```python
from build123d import *

# Parameters (mm, degrees)
SKETCH1_W                = 304.8
SKETCH1_H                = 304.8
BOSS_EXTRUDE1_DEPTH      = 5.334
SKETCH2_W                = 6.35
SKETCH2_H                = 101.6
CUT_EXTRUDE1_DEPTH       = 216.592141684
SKETCH26_W               = 11.599333334
SKETCH26_H               = 5.334
SKETCH26_W_2             = 5.334
SKETCH26_H_2             = 19.05
CUT_EXTRUDE11_DEPTH      = 216.592141684
SKETCH27_W               = 11.599333334
SKETCH27_H               = 5.334
SKETCH27_W_2             = 5.334
SKETCH27_H_2             = 19.05
CUT_EXTRUDE12_DEPTH      = 216.592141684
SKETCH29_W               = 304.8
SKETCH29_H               = 24.084758951
CUT_EXTRUDE13_DEPTH      = 216.592141684
SKETCH31_R               = 1.374999997
CUT_EXTRUDE15_DEPTH      = 216.592141684
SKETCH32_R               = 1.25
CUT_EXTRUDE16_DEPTH      = 216.592141684
SKETCH34_R               = 1.249249953
SKETCH34_R_2             = 1.249999995
SKETCH34_R_3             = 1.252496274
SKETCH34_R_4             = 1.251959019
CUT_EXTRUDE18_DEPTH      = 216.592141684
SKETCH38_R               = 1.248199844
SKETCH38_R_2             = 1.253619174
SKETCH38_R_3             = 1.25252158
SKETCH38_R_4             = 1.237868742
CUT_EXTRUDE22_DEPTH      = 216.592141684
SKETCH40_W               = 304.8
SKETCH40_H               = 5.334
BOSS_EXTRUDE2_DEPTH      = 76.2
SKETCH41_R               = 2.778125
CUT_EXTRUDE24_DEPTH      = 275.794780802
CUT_EXTRUDE25_DEPTH      = 275.794780802
CUT_EXTRUDE25_DEPTH_BACK = 275.794780802
SKETCH42_R               = 1.246523933
SKETCH42_R_2             = 1.251934436
SKETCH42_R_3             = 1.248703554
SKETCH42_R_4             = 1.245581387
SKETCH44_W               = 16.476980096
SKETCH44_H               = 3.5
SKETCH44_W_2             = 19.633145944
SKETCH44_H_2             = 3.596708667
CUT_EXTRUDE27_DEPTH      = 275.794780802
SKETCH45_W               = 20.354162164
SKETCH45_H               = 8.066046325
SKETCH45_W_2             = 20.554982424
SKETCH45_H_2             = 7.688212903
SKETCH45_H_3             = 7.652166289
SKETCH45_W_3             = 23.136298987
SKETCH45_H_4             = 7.272580335
CUT_EXTRUDE28_DEPTH      = 275.794780802
SKETCH46_W               = 304.8
SKETCH46_H               = 5.334
BOSS_EXTRUDE3_DEPTH      = 50.8
SKETCH47_R               = 9.778477959
SKETCH47_R_2             = 6.35205685
CUT_EXTRUDE29_DEPTH      = 275.794780802
SKETCH49_W               = 5.334
SKETCH49_H               = 19.05
SKETCH49_H_2             = 20.295839927
CUT_EXTRUDE30_DEPTH      = 275.794780802
SKETCH52_R               = 5.113702669
SKETCH52_R_2             = 5.177907844
CUT_EXTRUDE33_DEPTH      = 275.794780802


with BuildPart() as part:
    # Sketch1 → Boss-Extrude1 (new body)
    with BuildSketch(Plane.XY):
        Rectangle(SKETCH1_W, SKETCH1_H)
    extrude(amount=BOSS_EXTRUDE1_DEPTH)

    # Sketch2 → Cut-Extrude1 (cut, through all)
    with BuildSketch(Plane(origin=(0, 0, 0), x_dir=(-1, 0, 0), z_dir=(0, 0, -1))):
        with Locations((149.225, -63.5)):
            Rectangle(SKETCH2_W, SKETCH2_H)
        with Locations((-149.225, -63.5)):
            Rectangle(SKETCH2_W, SKETCH2_H)
    extrude(amount=-CUT_EXTRUDE1_DEPTH, mode=Mode.SUBTRACT)

    # Sketch26 → Cut-Extrude11 (cut, through all)
    with BuildSketch(Plane.XY.offset(5.334)):
        with Locations((-126.111, -89.408)):
            Rectangle(SKETCH26_W, SKETCH26_H)
        with Locations((-111.379, -63.5)):
            Rectangle(SKETCH26_W_2, SKETCH26_H_2)
        with Locations((-126.111, -37.592)):
            Rectangle(SKETCH26_W, SKETCH26_H)
        with Locations((-140.843, -63.5)):
            Rectangle(SKETCH26_W_2, SKETCH26_H_2)
    extrude(amount=-CUT_EXTRUDE11_DEPTH, mode=Mode.SUBTRACT)

    # Sketch27 → Cut-Extrude12 (cut, through all)
    with BuildSketch(Plane.XY.offset(5.334)):
        with Locations((126.111, -89.408)):
            Rectangle(SKETCH27_W, SKETCH27_H)
        with Locations((111.379, -63.5)):
            Rectangle(SKETCH27_W_2, SKETCH27_H_2)
        with Locations((126.111, -37.592)):
            Rectangle(SKETCH27_W, SKETCH27_H)
        with Locations((140.843, -63.5)):
            Rectangle(SKETCH27_W_2, SKETCH27_H_2)
    extrude(amount=-CUT_EXTRUDE12_DEPTH, mode=Mode.SUBTRACT)

    # Sketch29 → Cut-Extrude13 (cut, through all)
    with BuildSketch(Plane(origin=(0, 0, 0), x_dir=(-1, 0, 0), z_dir=(0, 0, -1))):
        with Locations((0, -140.357620525)):
            Rectangle(SKETCH29_W, SKETCH29_H)
    extrude(amount=-CUT_EXTRUDE13_DEPTH, mode=Mode.SUBTRACT)

    # Sketch31 → Cut-Extrude15 (cut, through all)
    with BuildSketch(Plane(origin=(0, 0, 0), x_dir=(-1, 0, 0), z_dir=(0, 0, -1))):
        with Locations((-94.072328828, 102.688814533)):
            Circle(SKETCH31_R)
        with Locations((-45.074194598, 103.116414773)):
            Circle(SKETCH31_R)
        with Locations((-93.566189769, 44.691022995)):
            Circle(SKETCH31_R)
        with Locations((-44.568055539, 45.118623235)):
            Circle(SKETCH31_R)
    extrude(amount=-CUT_EXTRUDE15_DEPTH, mode=Mode.SUBTRACT)

    # Sketch32 → Cut-Extrude16 (cut, through all)
    with BuildSketch(Plane(origin=(0, 0, 0), x_dir=(-1, 0, 0), z_dir=(0, 0, -1))):
        with Locations((-125.781887437, 64.718548335)):
            Circle(SKETCH32_R)
        with Locations((-141.021887437, 64.718548335)):
            Circle(SKETCH32_R)
        with Locations((-141.021887437, 43.128548335)):
            Circle(SKETCH32_R)
        with Locations((-125.781887437, 43.128548335)):
            Circle(SKETCH32_R)
    extrude(amount=-CUT_EXTRUDE16_DEPTH, mode=Mode.SUBTRACT)

    # Sketch34 → Cut-Extrude18 (cut, through all)
    with BuildSketch(Plane(origin=(0, 0, 0), x_dir=(-1, 0, 0), z_dir=(0, 0, -1))):
        with Locations((-75.859031626, -85.661481109)):
            Circle(SKETCH34_R)
        with Locations((-76.178771886, -122.30008597)):
            Circle(SKETCH34_R_2)
        with Locations((-19.220652784, -122.797151945)):
            Circle(SKETCH34_R_3)
        with Locations((-18.900912524, -86.158547084)):
            Circle(SKETCH34_R_4)
    extrude(amount=-CUT_EXTRUDE18_DEPTH, mode=Mode.SUBTRACT)

    # Sketch38 → Cut-Extrude22 (cut, through all)
    with BuildSketch(Plane(origin=(0, 0, 0), x_dir=(-1, 0, 0), z_dir=(0, 0, -1))):
        with Locations((43.524965306, -22.819488401)):
            Circle(SKETCH38_R)
        with Locations((-11.972921424, -22.335165681)):
            Circle(SKETCH38_R_2)
        with Locations((-12.457244144, -77.833052411)):
            Circle(SKETCH38_R_3)
        with Locations((43.040642586, -78.317375131)):
            Circle(SKETCH38_R_4)
    extrude(amount=-CUT_EXTRUDE22_DEPTH, mode=Mode.SUBTRACT)

    # Sketch40 → Boss-Extrude2 (add)
    with BuildSketch(Plane(origin=(0, 152.4, 0), x_dir=(1, 0, 0), z_dir=(0, 1, 0))):
        with Locations((0, -2.667)):
            Rectangle(SKETCH40_W, SKETCH40_H)
    extrude(amount=BOSS_EXTRUDE2_DEPTH)

    # Sketch41 → Cut-Extrude24 (cut, through all)
    with BuildSketch(Plane(origin=(0, 0, 0), x_dir=(-1, 0, 0), z_dir=(0, 0, -1))):
        with Locations((-27.760706508, 199.901266022)):
            Circle(SKETCH41_R)
        with Locations((27.760706508, 197.764889884)):
            Circle(SKETCH41_R)
    extrude(amount=-CUT_EXTRUDE24_DEPTH, mode=Mode.SUBTRACT)

    # Sketch42 → Cut-Extrude25 (cut, two sides: drawn at the far end of the back side and taken through both)
    with BuildSketch(Plane(origin=(0, 0, 0), x_dir=(-1, 0, 0), z_dir=(0, 0, -1)).offset(-CUT_EXTRUDE25_DEPTH_BACK)):
        with Locations((-40.428890621, -22.652536653)):
            Circle(SKETCH42_R)
        with Locations((-107.546334897, -23.238261716)):
            Circle(SKETCH42_R_2)
        with Locations((-107.954736758, 23.559956283)):
            Circle(SKETCH42_R_3)
        with Locations((-40.837292482, 24.145681346)):
            Circle(SKETCH42_R_4)
    extrude(amount=CUT_EXTRUDE25_DEPTH + CUT_EXTRUDE25_DEPTH_BACK, mode=Mode.SUBTRACT)

    # Sketch44 → Cut-Extrude27 (cut, through all)
    with BuildSketch(Plane(origin=(0, 0, 0), x_dir=(-1, 0, 0), z_dir=(0, 0, -1))):
        with Locations((76.712846496, -123.491430997)):
            Rectangle(SKETCH44_W, SKETCH44_H)
        with Locations((76.712846496, -94.591430997)):
            Rectangle(SKETCH44_W, SKETCH44_H)
        with Locations((45.782293013, -123.539785331)):
            Rectangle(SKETCH44_W_2, SKETCH44_H_2)
        with Locations((45.782293013, -94.688139664)):
            Rectangle(SKETCH44_W_2, SKETCH44_H)
    extrude(amount=-CUT_EXTRUDE27_DEPTH, mode=Mode.SUBTRACT)

    # Sketch45 → Cut-Extrude28 (cut, through all)
    with BuildSketch(Plane(origin=(0, 0, 0), x_dir=(-1, 0, 0), z_dir=(0, 0, -1))):
        with Locations((95.443302682, 192.238942395)):
            Rectangle(SKETCH45_W, SKETCH45_H)
        with Locations((52.047470718, 192.427859106)):
            Rectangle(SKETCH45_W_2, SKETCH45_H_2)
        with Locations((52.047470716, 121.434632147)):
            Rectangle(SKETCH45_W_2, SKETCH45_H_3)
        with Locations((96.834371094, 121.24483917)):
            Rectangle(SKETCH45_W_3, SKETCH45_H_4)
    extrude(amount=-CUT_EXTRUDE28_DEPTH, mode=Mode.SUBTRACT)

    # Sketch46 → Boss-Extrude3 (add)
    with BuildSketch(Plane.XZ.offset(128.315241049)):
        with Locations((0, 2.667)):
            Rectangle(SKETCH46_W, SKETCH46_H)
    extrude(amount=BOSS_EXTRUDE3_DEPTH)

    # Sketch47 → Cut-Extrude29 (cut, through all)
    with BuildSketch(Plane(origin=(0, 0, 0), x_dir=(-1, 0, 0), z_dir=(0, 0, -1))):
        with Locations((-131.017495066, 88.21224972)):
            Circle(SKETCH47_R)
        with Locations((-137.650958824, 18.755982137)):
            Circle(SKETCH47_R_2)
    extrude(amount=-CUT_EXTRUDE29_DEPTH, mode=Mode.SUBTRACT)

    # Sketch49 → Cut-Extrude30 (cut, through all)
    with BuildSketch(Plane.XY.offset(5.334)):
        with Locations((-27.846255785, 9.907194542)):
            Rectangle(SKETCH49_W, SKETCH49_H)
        with Locations((-107.982405159, 9.907194542)):
            Rectangle(SKETCH49_W, SKETCH49_H)
        with Locations((-107.982405159, 51.068016377)):
            Rectangle(SKETCH49_W, SKETCH49_H_2)
        with Locations((-107.982405159, 100.839194542)):
            Rectangle(SKETCH49_W, SKETCH49_H)
        with Locations((-27.846255785, 100.839194542)):
            Rectangle(SKETCH49_W, SKETCH49_H)
        with Locations((-27.846255785, 51.068016377)):
            Rectangle(SKETCH49_W, SKETCH49_H_2)
    extrude(amount=-CUT_EXTRUDE30_DEPTH, mode=Mode.SUBTRACT)

    # Sketch52 → Cut-Extrude33 (cut, through all)
    with BuildSketch(Plane(origin=(0, 0, 0), x_dir=(-1, 0, 0), z_dir=(0, 0, -1))):
        with Locations((-57.021451744, 149.159143491)):
            Circle(SKETCH52_R)
        with Locations((-57.021451744, 166.299522531)):
            Circle(SKETCH52_R_2)
    extrude(amount=-CUT_EXTRUDE33_DEPTH, mode=Mode.SUBTRACT)


solid = part.part
```
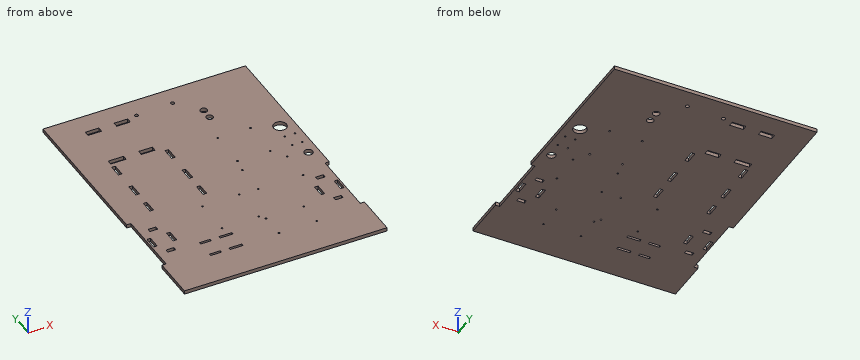
Build history of the part. All positions in model axes, mm. Round coordinates to 2 decimals unless told otherwise and drop trailing zeros. Order: outer loops, then holes, each group sorted by start corner. A loop starts at its lowest first (then second) coordinate and runs counter-clockwise, first axis right, second up. Notation, with made-up numbers: (-35.75, 80) -> (7.25, 80) arc R33 ccw to (7.25, 114) -> close; hole circle Ø1 at (-5, 15). An arc over 180 degrees is marked (long way). Answer in a Markdown table with one row per item.
1) Pin check, flat tips, straight feed: P1, Ø8.5, axis at x = 57.02, y = 166.3, coming from the +Z side; P2, Ø1.6, axis at y = -88.5, z = 2.5, coming from the +X side. Stop position of each tip, or through.
Values:
| item | result |
|---|---|
| P1 | through |
| P2 | x = 146.05 |
2) Band-saw the part on B-B on x = -50. Give the cut face in (y, z).
Values:
| item | result |
|---|---|
| outline | (-179.12, 0) -> (-125.34, 0) -> (-125.34, 5.33) -> (-179.12, 5.33) -> close; (-121.74, 0) -> (-96.44, 0) -> (-96.44, 5.33) -> (-121.74, 5.33) -> close; (-92.94, 0) -> (117.61, 0) -> (117.61, 5.33) -> (-92.94, 5.33) -> close; (125.26, 0) -> (188.58, 0) -> (188.58, 5.33) -> (125.26, 5.33) -> close; (196.27, 0) -> (228.6, 0) -> (228.6, 5.33) -> (196.27, 5.33) -> close |
3) Band-saw the part on C-C on z = 1.15. Give the number of separate pieces and of enclosed holes in the cut face, and give its area (3 significant figures).
Values:
| item | result |
|---|---|
| separate pieces | 1 |
| enclosed holes | 48 |
| area | 120,000 mm2 |
4) Wall check: L1, parallel to Y at x = -120.5, z = 2.8 (3 decimals); L2, parallel to Y at x = -81.5, z = 2.45; L3, parallel to Y at x = -110, z = 5.1 (3 decimals). Give the ranges that are in metal, low to high.
Values:
| item | result |
|---|---|
| L1 | -179.115 to -92.075, -86.741 to -40.259, -34.925 to 228.6 |
| L2 | -179.12 to -125.24, -121.74 to -96.34, -92.84 to 228.6 |
| L3 | -179.115 to -73.025, -53.975 to 0.382, 19.432 to 40.92, 61.216 to 91.314, 110.364 to 228.6 |
5) Band-saw the part on A-A on y = -63. Give the cut face in (x, z).
Values:
| item | result |
|---|---|
| outline | (-146.05, 0) -> (-143.51, 0) -> (-143.51, 5.33) -> (-146.05, 5.33) -> close; (-138.18, 0) -> (-114.05, 0) -> (-114.05, 5.33) -> (-138.18, 5.33) -> close; (-108.71, 0) -> (108.71, 0) -> (108.71, 5.33) -> (-108.71, 5.33) -> close; (114.05, 0) -> (138.18, 0) -> (138.18, 5.33) -> (114.05, 5.33) -> close; (143.51, 0) -> (146.05, 0) -> (146.05, 5.33) -> (143.51, 5.33) -> close |
